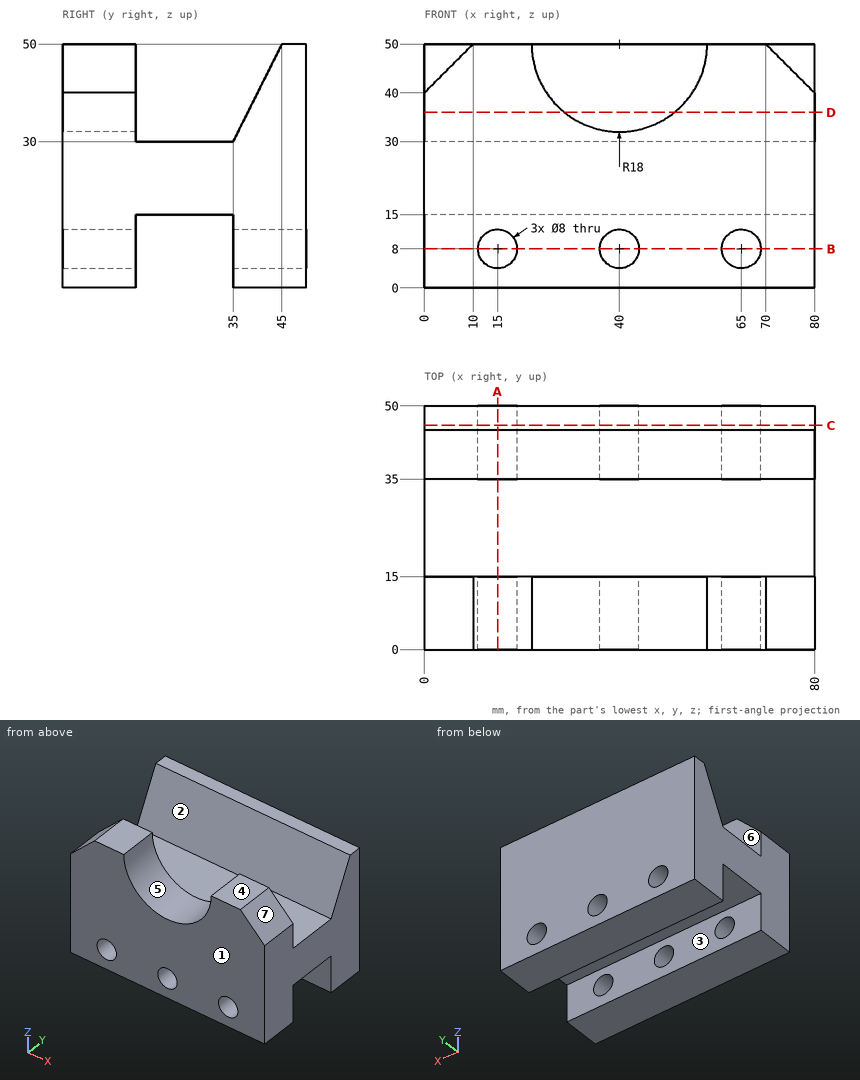
Input: dimensioned drawing with shaded views. Units: mm. Origin: part minimum x, y, z. A direction names the side the tool comes from. Coordinates: 2 decimals unless noted, no trailing zeros. Order: outer loops, then holes, each group sorted by start corner. A loop starts at its lowest first (then second) coordinate and runs counter-clockwise, first axis right, second up. Notation, with made-up numbers: (54.25, 73) - (84.25, 73) arc R17 cw to (84.25, 85) - close; hole circle Ø5 at (-14, 14.25). An arc over 180 degrees is marked (long way). One line per item, written item: value.
1) Reachability of the marked faces 5, 6 and 7 from +Z, -Z, +X, -X, +Y, -Y: full face, straight path, thin tool, end or side. Return the list, or none.
Computed values:
face 5: +Z, -Y
face 6: +Z, +X, -X
face 7: +Z, +X, -Y
2) Ray query, line 1 (Y direction, x = 47.5, z = 8); line 2 (Z direction, x = 15, y = 5); line 3 (Z direction, x = 20, y = 22.5). Return the intervals inside material, ascending. Write a range as [from, to].
Computed values:
line 1: y = [0, 15], [35, 50]
line 2: z = [0, 4], [12, 50]
line 3: z = [15, 30]
3) Mould query, pull axis Y, two halves, no side actions, for the marked faces 1, 2, 3 and 4. Classes: released by +Y, released by -Y, zero draft, split by the parting line, or undercut.
Computed values:
face 1: released by -Y
face 2: undercut
face 3: undercut
face 4: zero draft
4) Contact query for flat-ended pins moving along their axis: pin 1 (13 mm diameter, centred on x = 15, z = 8, fed in from -Y); pin 2 (1.5 mm diameter, centred on x = 40, y = 21.5, fed in from -Z); pin 3 (10 mm diameter, centred on x = 41, y = 28, fed in from +Z). Output: stop coordinate, or through.
Computed values:
pin 1: stops at y = 0
pin 2: stops at z = 15
pin 3: stops at z = 30
5) Cut plane A-A on x = 15. Output: boundary loops of the cut face in (y, z), plus the area to 3 significant figures.
Computed values:
outline: (0, 0) - (15, 0) - (15, 4) - (0, 4) - close; (0, 12) - (15, 12) - (15, 15) - (35, 15) - (35, 12) - (50, 12) - (50, 50) - (45, 50) - (35, 30) - (15, 30) - (15, 50) - (0, 50) - close; (35, 0) - (50, 0) - (50, 4) - (35, 4) - close
area: 1,460 mm^2
6) Cut plane D-D on z = 36. Output: boundary loops of the cut face in (x, y).
Computed values:
outline: (0, 0) - (28.69, 0) - (28.69, 15) - (0, 15) - close; (0, 38) - (80, 38) - (80, 50) - (0, 50) - close; (51.31, 0) - (80, 0) - (80, 15) - (51.31, 15) - close
7) Cut plane B-B on z = 8. State how many separate pieces and enclosed holes the cut face has, plus the area to 3 significant figures.
Computed values:
separate pieces: 8
enclosed holes: 0
area: 1,680 mm^2
8) Cut plane C-C on y = 46. Output: boundary loops of the cut face in (x, z), plus the area to 3 significant figures.
Computed values:
outline: (0, 0) - (80, 0) - (80, 50) - (0, 50) - close; hole circle Ø8 at (15, 8); hole circle Ø8 at (40, 8); hole circle Ø8 at (65, 8)
area: 3,850 mm^2
